from build123d import *

# Parameters (mm, degrees)
F3_DEPTH = 5


# Not quite as in the source:
# - after a boolean that leaves OpenCascade's solid faulty, fix() repairs it


with BuildPart() as f1:
    # F0 (on Front) → F1 (revolve)
    with BuildSketch(Plane.XZ):
        with BuildLine():
            Line((0, 40), (0, 0))
            Line((0, 0), (9, 0))
            ThreePointArc((9, 0), (12, 3), (9, 6))
            ThreePointArc((9, 6), (12, 9), (9, 12))
            Line((9, 12), (6.4358137697, 34.5418713987))
            Line((6.4358137697, 34.5418713987), (12.6394796214, 36.6926416755))
            Line((12.6394796214, 36.6926416755), (12.6394796214, 40))
            Line((12.6394796214, 40), (0, 40))
        make_face()
    revolve(axis=Axis((0, 0, 20), (0, 0, -1)))

    # F2 (on face) → F3 (join)
    with BuildSketch(Plane.XY.offset(40)):
        with BuildLine():
            ThreePointArc((-8.94427191, 1), (-8.3149157926, 3.4441508913), (-7.0316621015, 5.6174485392))
            Line((-7.0316621015, 5.6174485392), (-9.6165524738, 8.2023389114))
            ThreePointArc((-9.6165524738, 8.2023389114), (-11.6773565238, 4.8369194448), (-12.5998589317, 1))
            Line((-12.5998589317, 1), (-8.94427191, 1))
        make_face()
        with BuildLine():
            ThreePointArc((-1, 12.5998589317), (-4.8369194448, 11.6773565238), (-8.2023389114, 9.6165524738))
            Line((-8.2023389114, 9.6165524738), (-5.6174485392, 7.0316621015))
            ThreePointArc((-5.6174485392, 7.0316621015), (-3.4441508913, 8.3149157926), (-1, 8.94427191))
            Line((-1, 8.94427191), (-1, 12.5998589317))
        make_face()
        with BuildLine():
            ThreePointArc((8.2023389114, 9.6165524738), (4.8369194448, 11.6773565238), (1, 12.5998589317))
            Line((1, 12.5998589317), (1, 8.94427191))
            ThreePointArc((1, 8.94427191), (3.4441508913, 8.3149157926), (5.6174485392, 7.0316621015))
            Line((5.6174485392, 7.0316621015), (8.2023389114, 9.6165524738))
        make_face()
        with BuildLine():
            ThreePointArc((12.5998589317, 1), (11.6773565238, 4.8369194448), (9.6165524738, 8.2023389114))
            Line((9.6165524738, 8.2023389114), (7.0316621015, 5.6174485392))
            ThreePointArc((7.0316621015, 5.6174485392), (8.3149157926, 3.4441508913), (8.94427191, 1))
            Line((8.94427191, 1), (12.5998589317, 1))
        make_face()
        with BuildLine():
            Line((7.0316621015, -5.6174485392), (9.6165524738, -8.2023389114))
            ThreePointArc((9.6165524738, -8.2023389114), (11.6773565238, -4.8369194448), (12.5998589317, -1))
            Line((12.5998589317, -1), (8.94427191, -1))
            ThreePointArc((8.94427191, -1), (8.3149157926, -3.4441508913), (7.0316621015, -5.6174485392))
        make_face()
        with BuildLine():
            Line((1, -8.94427191), (1, -12.5998589317))
            ThreePointArc((1, -12.5998589317), (4.8369194448, -11.6773565238), (8.2023389114, -9.6165524738))
            Line((8.2023389114, -9.6165524738), (5.6174485392, -7.0316621015))
            ThreePointArc((5.6174485392, -7.0316621015), (3.4441508913, -8.3149157926), (1, -8.94427191))
        make_face()
        with BuildLine():
            Line((-5.6174485392, -7.0316621015), (-8.2023389114, -9.6165524738))
            ThreePointArc((-8.2023389114, -9.6165524738), (-4.8369194448, -11.6773565238), (-1, -12.5998589317))
            Line((-1, -12.5998589317), (-1, -8.94427191))
            ThreePointArc((-1, -8.94427191), (-3.4441508913, -8.3149157926), (-5.6174485392, -7.0316621015))
        make_face()
        with BuildLine():
            Line((-8.94427191, -1), (-12.5998589317, -1))
            ThreePointArc((-12.5998589317, -1), (-11.6773565238, -4.8369194448), (-9.6165524738, -8.2023389114))
            Line((-9.6165524738, -8.2023389114), (-7.0316621015, -5.6174485392))
            ThreePointArc((-7.0316621015, -5.6174485392), (-8.3149157926, -3.4441508913), (-8.94427191, -1))
        make_face()
    extrude(amount=F3_DEPTH)

    add(f1.part.fix(), mode=Mode.REPLACE)


solid = f1.part
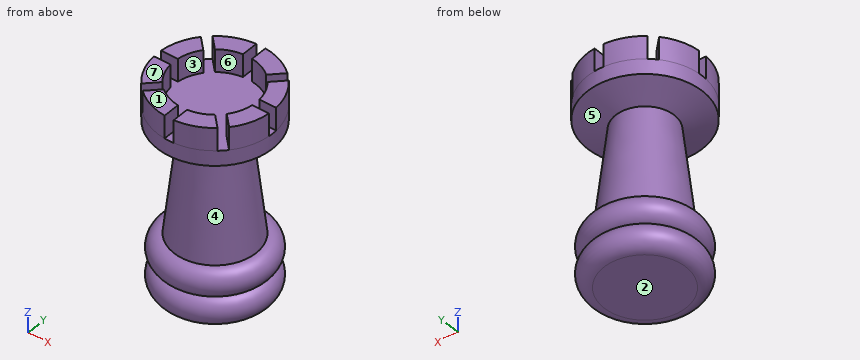
The listing builds one solid part. Answer for the finished solid, in the listing's coordinates (mm). Face numbers are marked on the shaded views. A direction names the side the tool comes from. Give positions to 0.01 mm unless a question says otherwise; leave off trailing zeros. Loops run counter-clockwise (first coordinate to the right, second up) from the corner with the lowest first, then second, coordinate; pieces in that order, holes last. Notation, with made-up numbers: (12, 66.5) - (64, 66.5) arc R20 cw to (64, 71.5) - close; hole circle Ø4 at (73.25, 36). An arc over 180 degrees is marked (long way). Answer as a JSON object with one key per item and string values.
1. A cutting plane is placed at C-C (z = 5). Write down the section's boundary in (x, y), then the cut area to 3 significant figures.
Determined:
{"outline": "circle Ø22.47 at (0, 0)", "area": "397 mm²"}
2. A cutting plane is placed at A-A (x = 0). Write down the section's boundary in (y, z).
Determined:
{"outline": "(-12.64, 36.69) - (-6.44, 34.54) - (-9, 12) arc R3 ccw to (-9, 6) arc R3 ccw to (-9, 0) - (9, 0) arc R3 ccw to (9, 6) arc R3 ccw to (9, 12) - (6.44, 34.54) - (12.64, 36.69) - (12.64, 40) - (-12.64, 40) - close"}
3. A cutting plane is placed at D-D (x = -10.75). Give the number of separate pieces and of enclosed holes in the cut face, then the cut area to 3 significant figures.
Determined:
{"separate pieces": "3", "enclosed holes": "0", "area": "190 mm²"}
4. Find the intervals of material crossed by L1, parallel to Z at x = -1.25, y = 10.5; L2, parallel to Z at x = 6, y = -8; L3, parallel to Z at x = -3.75, y = 3.75, in increasing order. Write a range as [from, to].
Determined:
{"L1": "[0.45, 5.55], [6.45, 11.55], [35.98, 45]", "L2": "[0.17, 5.83], [6.17, 11.83], [35.78, 45]", "L3": "[0, 40]"}
5. Flat-ended cylindrical pins translate along their axes: pin 1 Ø3 at (x, z) = (10.5, 42) entering from +Y; pin 2 Ø3 at (x, z) = (-10, 43.5) entering from -Y; pin 3 Ø1 at (y, z) = (6, 22) entering from +X (3 decimals); pin 4 Ø1.5 at (x, z) = (-9, 32.5) entering from -Y. Find the tip coordinate at first contact, or state that the pin passes through.
Determined:
{"pin 1": "y = 8.2", "pin 2": "y = -8.2", "pin 3": "x = 5.625", "pin 4": "through"}
6. For a pull along Z with two mould halves and no side action, classify the marked faces 1, 2, 3 and 4 as pulls with the +Z half, pulls with the -Z half, needs draft (parallel to the pull), parting line crosses it, or undercut.
Determined:
{"face 1": "pulls with the +Z half", "face 2": "pulls with the -Z half", "face 3": "needs draft", "face 4": "undercut"}
7. For the marked faces 5, 6 and 7, determine the directions among +Z, -Z, +X, -X, +Y, -Y from which every point of the face is accessible in a straight line to the end or side of a thin tool.
Determined:
{"face 5": "none", "face 6": "+Z", "face 7": "+Z, +X, -X, +Y, -Y"}
